Input: part model. Units: mm. Frame: model coordinates. Face numbers are marked on the shaded views. A direction names the side the tool comes from. Round coordinates to 2 decimals unless told otherwise and drop trailing zeros. Order: outer loops, then holes, each group sorted by start corner. A loop starts at its lowest first (then second) coordinate and runs counter-clockwise, first axis right, second up.
Item 1: Cut plane B-B on x = 0. Output: boundary loops of the cut face in (y, z).
Item 2: Cut plane D-D on x = 5.75. Output: boundary loops of the cut face in (y, z).
Item 3: Cut plane C-C on z = 6.5. Output: boundary loops of the cut face in (x, y), then the cut area to 3 significant figures.
Item 4: Cut plane A-A on y = 0. Output: boundary loops of the cut face in (x, z), then the cut area to 3 significant figures.
Item 5: Line query: L1, parallel to X at y = 0, z = 41.5; L2, parallel to Z at x = 3.5, y = -5.75; L3, parallel to Z at x = 0, y = -1. Output: solid intervals per line, ascending.
Item 6: Reachability of the marked faces 1 and 2 from +Z, -Z, +X, -X, +Y, -Y: full face, straight path, thin tool, end or side. Return the list, or none.
Item 7: First-contact query: pin 1 (6 mm diameter, centred on y = 0, z = 13.5, fed in from -X); pin 2 (0.5 mm diameter, centred on y = 6.5, z = 19, fed in from -X); pin 3 (4 mm diameter, centred on x = 0, z = 17.5, fed in from -Y). Flat tips, straight axial feed; report the tip coordinate or a pass-through.
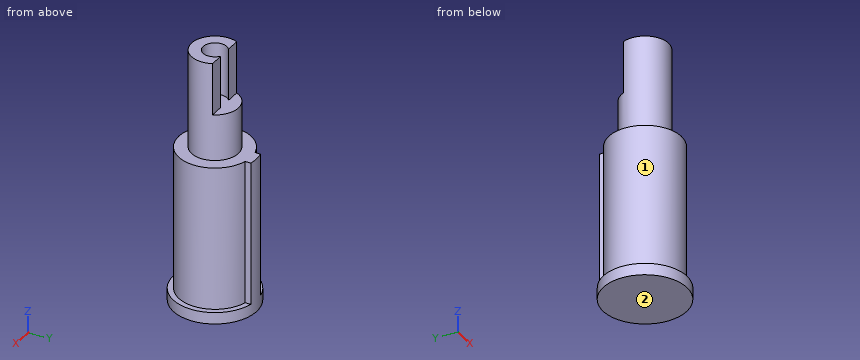
Autodesk Inventor part; units mm, degrees
ref_plane "YZ Plane" through (0, 0, 0) normal (1, 0, 0) x (0, 1, 0)
ref_plane "XZ Plane" through (0, 0, 0) normal (0, 1, 0) x (-1, 0, 0)
ref_plane "XY Plane" through (0, 0, 0) normal (0, 0, 1) x (1, 0, 0)
sketch "スケッチ1" plane through (0, 0, 0) normal (0, 0, 1) x (1, 0, 0)
  circle A0 centre (0, 0) radius 7.2
  dimension "d0" = 14.4
extrude "押し出し1" add sketch "スケッチ1" along normal blind 2
sketch "スケッチ2" plane through (0, 0, 2) normal (0, 0, 1) x (1, 0, 0)
  circle A0 centre (0, 0) radius 6.25
  line L0 (-1.5, 6.0673) -> (-1.5, 7.042)
  circle A1 centre (0, 0) radius 7.2
  line L1 (1.5, 7.042) -> (1.5, 6.0673)
  dimension "d3" = 12.5
  dimension "d6" = 1.5
  dimension "d7" = 1.5
extrude "押し出し2" add sketch "スケッチ2" along normal blind 24.8 contours A0 | A0 L0 A1 L1 picked at (1.1681, 6.4463)
sketch "スケッチ3" plane through (0, 0, 26.8) normal (0, 0, 1) x (1, 0, 0)
  circle A0 centre (0, 0) radius 4.05
  circle A1 centre (0, 0) radius 2.05
  line L0 (-1.2, 1.6621) -> (1.2, 1.6621)
  line L1 (-1.2, 1.6621) -> (-3.6932, 1.6621)
  line L2 (1.2, 1.6621) -> (3.6932, 1.6621)
  dimension "d8" = 8.1
  dimension "d9" = 4.1
  dimension "d10" = 2.4
extrude "押し出し3" add sketch "スケッチ3" along normal blind 17 contours A0 L1 A1 L2 picked at (3.3454, -0.3178)
extrude "押し出し4" add sketch "スケッチ3" along normal blind 8 contours L2 A1 L1 A0 | L0 A1 | A1 L0 picked at (-2.7038, 1.9277)
properties part number "SU22_3DP_EncorderUnit_Bar_sn" material "ABS プラスチック"
From the geometry:
1. outline: (-7.2, 0) - (7.2, 0) - (7.2, 26.8) - (4.05, 26.8) - (4.05, 34.8) - (-2.05, 34.8) - (-2.05, 43.8) - (-4.05, 43.8) - (-4.05, 26.8) - (-6.25, 26.8) - (-6.25, 2) - (-7.2, 2) - close
2. outline: (-4.33, 0) - (4.33, 0) - (4.33, 2) - (2.45, 2) - (2.45, 26.8) - (-2.45, 26.8) - (-2.45, 2) - (-4.33, 2) - close
3. outline: (-1.5, 6.07) arc R6.25 ccw (long way) to (1.5, 6.07) - (1.5, 7.04) arc R7.2 ccw to (-1.5, 7.04) - close
3. area: 126 mm2
4. outline: (-7.2, 0) - (7.2, 0) - (7.2, 2) - (6.25, 2) - (6.25, 26.8) - (4.05, 26.8) - (4.05, 43.8) - (2.05, 43.8) - (2.05, 34.8) - (-2.05, 34.8) - (-2.05, 43.8) - (-4.05, 43.8) - (-4.05, 26.8) - (-6.25, 26.8) - (-6.25, 2) - (-7.2, 2) - close
4. area: 440 mm2
5. L1: x = -4.05 to -2.05, 2.05 to 4.05
5. L2: z = 0 to 2
5. L3: z = 0 to 34.8
6. face 1: +Z
6. face 2: -Z, +X, -X, +Y, -Y
7. pin 1: stops at x = -6.25
7. pin 2: stops at x = -1.5
7. pin 3: stops at y = -6.25
